from build123d import *

# Parameters (mm, degrees)
SKETCH1_R           = 35
SKETCH1_R_2         = 17.3
BOSS_EXTRUDE1_DEPTH = 2.5
BOSS_EXTRUDE2_START = 2
SKETCH3_R           = 35
SKETCH3_R_2         = 18.6
BOSS_EXTRUDE2_DEPTH = 2
BOSS_EXTRUDE3_START = 2
SKETCH4_R           = 35
SKETCH4_R_2         = 22.3
BOSS_EXTRUDE3_DEPTH = 2
CUT_EXTRUDE1_REACH  = 51.922
SKETCH6_R           = 1.3
BOSS_EXTRUDE6_START = -10
SKETCH7_R           = 35
SKETCH7_W           = 54
SKETCH7_H           = 70
BOSS_EXTRUDE6_DEPTH = 10
SKETCH8_W           = 7
SKETCH8_H           = 70
CUT_EXTRUDE3_DEPTH  = 3
CUT_EXTRUDE4_REACH  = 133.476
SKETCH10_R          = 2.8


with BuildPart() as part:
    # Sketch1 → Boss-Extrude1 (new body)
    with BuildSketch(Plane(origin=(0, 0, 0), x_dir=(1, 0, 0), z_dir=(0, 1, 0))):
        with Locations(Location((0, 0, 0), (0, 0, 270))):
            Circle(SKETCH1_R)
        with Locations(Location((0, 0, 0), (0, 0, 270))):
            Circle(SKETCH1_R_2, mode=Mode.SUBTRACT)
    extrude(amount=BOSS_EXTRUDE1_DEPTH)

    # Sketch3 → Boss-Extrude2 (add)
    with BuildSketch(Plane.XZ.offset(BOSS_EXTRUDE2_START)):
        with Locations(Location((0, 0, 0), (0, 0, 270))):
            Circle(SKETCH3_R)
        with Locations(Location((0, 0, 0), (0, 0, 270))):
            Circle(SKETCH3_R_2, mode=Mode.SUBTRACT)
    extrude(amount=-BOSS_EXTRUDE2_DEPTH)

    # Sketch4 → Boss-Extrude3 (add)
    with BuildSketch(Plane.XZ.offset(2).offset(BOSS_EXTRUDE3_START)):
        with Locations(Location((0, 0, 0), (0, 0, 270))):
            Circle(SKETCH4_R)
        with Locations(Location((0, 0, 0), (0, 0, 270))):
            Circle(SKETCH4_R_2, mode=Mode.SUBTRACT)
    extrude(amount=-BOSS_EXTRUDE3_DEPTH)

    # Sketch6 → Cut-Extrude1 (cut, up to next)
    with BuildSketch(Plane(origin=(0, 2.5, 0), x_dir=(1, 0, 0), z_dir=(0, 1, 0)), mode=Mode.PRIVATE) as cut_extrude1_sk1:
        with Locations(Location((0, 20.25, 0), (0, 0, 270))):
            Circle(SKETCH6_R)
    cut_extrude1_tool1 = extrude(cut_extrude1_sk1.sketch, amount=-CUT_EXTRUDE1_REACH, mode=Mode.PRIVATE) & part.part
    # Sketch6 → Cut-Extrude1 (cut, up to next)
    with BuildSketch(Plane(origin=(0, 2.5, 0), x_dir=(1, 0, 0), z_dir=(0, 1, 0)), mode=Mode.PRIVATE) as cut_extrude1_sk2:
        with Locations(Location((14.318912319, 14.318912319, 0), (0, 0, 270))):
            Circle(SKETCH6_R)
    cut_extrude1_tool2 = extrude(cut_extrude1_sk2.sketch, amount=-CUT_EXTRUDE1_REACH, mode=Mode.PRIVATE) & part.part
    # Sketch6 → Cut-Extrude1 (cut, up to next)
    with BuildSketch(Plane(origin=(0, 2.5, 0), x_dir=(1, 0, 0), z_dir=(0, 1, 0)), mode=Mode.PRIVATE) as cut_extrude1_sk3:
        with Locations(Location((20.25, 0, 0), (0, 0, 270))):
            Circle(SKETCH6_R)
    cut_extrude1_tool3 = extrude(cut_extrude1_sk3.sketch, amount=-CUT_EXTRUDE1_REACH, mode=Mode.PRIVATE) & part.part
    # Sketch6 → Cut-Extrude1 (cut, up to next)
    with BuildSketch(Plane(origin=(0, 2.5, 0), x_dir=(1, 0, 0), z_dir=(0, 1, 0)), mode=Mode.PRIVATE) as cut_extrude1_sk4:
        with Locations(Location((14.318912319, -14.318912319, 0), (0, 0, 270))):
            Circle(SKETCH6_R)
    cut_extrude1_tool4 = extrude(cut_extrude1_sk4.sketch, amount=-CUT_EXTRUDE1_REACH, mode=Mode.PRIVATE) & part.part
    # Sketch6 → Cut-Extrude1 (cut, up to next)
    with BuildSketch(Plane(origin=(0, 2.5, 0), x_dir=(1, 0, 0), z_dir=(0, 1, 0)), mode=Mode.PRIVATE) as cut_extrude1_sk5:
        with Locations(Location((0, -20.25, 0), (0, 0, 270))):
            Circle(SKETCH6_R)
    cut_extrude1_tool5 = extrude(cut_extrude1_sk5.sketch, amount=-CUT_EXTRUDE1_REACH, mode=Mode.PRIVATE) & part.part
    # Sketch6 → Cut-Extrude1 (cut, up to next)
    with BuildSketch(Plane(origin=(0, 2.5, 0), x_dir=(1, 0, 0), z_dir=(0, 1, 0)), mode=Mode.PRIVATE) as cut_extrude1_sk6:
        with Locations(Location((-14.318912319, -14.318912319, 0), (0, 0, 270))):
            Circle(SKETCH6_R)
    cut_extrude1_tool6 = extrude(cut_extrude1_sk6.sketch, amount=-CUT_EXTRUDE1_REACH, mode=Mode.PRIVATE) & part.part
    # Sketch6 → Cut-Extrude1 (cut, up to next)
    with BuildSketch(Plane(origin=(0, 2.5, 0), x_dir=(1, 0, 0), z_dir=(0, 1, 0)), mode=Mode.PRIVATE) as cut_extrude1_sk7:
        with Locations(Location((-20.25, 0, 0), (0, 0, 270))):
            Circle(SKETCH6_R)
    cut_extrude1_tool7 = extrude(cut_extrude1_sk7.sketch, amount=-CUT_EXTRUDE1_REACH, mode=Mode.PRIVATE) & part.part
    # Sketch6 → Cut-Extrude1 (cut, up to next)
    with BuildSketch(Plane(origin=(0, 2.5, 0), x_dir=(1, 0, 0), z_dir=(0, 1, 0)), mode=Mode.PRIVATE) as cut_extrude1_sk8:
        with Locations(Location((-14.318912319, 14.318912319, 0), (0, 0, 270))):
            Circle(SKETCH6_R)
    cut_extrude1_tool8 = extrude(cut_extrude1_sk8.sketch, amount=-CUT_EXTRUDE1_REACH, mode=Mode.PRIVATE) & part.part
    add(cut_extrude1_tool1.solids().sort_by_distance((0, 2.5, -20.25))[0], mode=Mode.SUBTRACT)
    add(cut_extrude1_tool2.solids().sort_by_distance((14.318912, 2.5, -14.318912))[0], mode=Mode.SUBTRACT)
    add(cut_extrude1_tool3.solids().sort_by_distance((20.25, 2.5, 0))[0], mode=Mode.SUBTRACT)
    add(cut_extrude1_tool4.solids().sort_by_distance((14.318912, 2.5, 14.318912))[0], mode=Mode.SUBTRACT)
    add(cut_extrude1_tool5.solids().sort_by_distance((0, 2.5, 20.25))[0], mode=Mode.SUBTRACT)
    add(cut_extrude1_tool6.solids().sort_by_distance((-14.318912, 2.5, 14.318912))[0], mode=Mode.SUBTRACT)
    add(cut_extrude1_tool7.solids().sort_by_distance((-20.25, 2.5, 0))[0], mode=Mode.SUBTRACT)
    add(cut_extrude1_tool8.solids().sort_by_distance((-14.318912, 2.5, -14.318912))[0], mode=Mode.SUBTRACT)

    # Sketch7 → Boss-Extrude6 (add)
    with BuildSketch(Plane(origin=(0, 2.5, 0), x_dir=(1, 0, 0), z_dir=(0, 1, 0)).offset(BOSS_EXTRUDE6_START)):
        Polygon((-45, 55), (99, 55), (119, 55), (119, -55), (99, -55), (-35, -55), (-45, -55), (-45, 35), align=None)
        with Locations(Location((0, 0, 0), (0, 0, 270))):
            Circle(SKETCH7_R, mode=Mode.SUBTRACT)
        with Locations((72, 0)):
            Rectangle(SKETCH7_W, SKETCH7_H, mode=Mode.SUBTRACT)
    extrude(amount=BOSS_EXTRUDE6_DEPTH)

    # Sketch8 → Cut-Extrude3 (cut)
    with BuildSketch(Plane.XZ.offset(7.5)):
        with Locations((102.5, 0)):
            Rectangle(SKETCH8_W, SKETCH8_H)
        with Locations((41.5, 0)):
            Rectangle(SKETCH8_W, SKETCH8_H)
    extrude(amount=-CUT_EXTRUDE3_DEPTH, mode=Mode.SUBTRACT)

    # Sketch10 → Cut-Extrude4 (cut, up to next)
    with BuildSketch(Plane(origin=(0, 2.5, 0), x_dir=(1, 0, 0), z_dir=(0, 1, 0)), mode=Mode.PRIVATE) as cut_extrude4_sk1:
        with Locations(Location((37, 45, 0), (0, 0, 270))):
            Circle(SKETCH10_R)
    cut_extrude4_tool1 = extrude(cut_extrude4_sk1.sketch, amount=-CUT_EXTRUDE4_REACH, mode=Mode.PRIVATE) & part.part
    # Sketch10 → Cut-Extrude4 (cut, up to next)
    with BuildSketch(Plane(origin=(0, 2.5, 0), x_dir=(1, 0, 0), z_dir=(0, 1, 0)), mode=Mode.PRIVATE) as cut_extrude4_sk2:
        with Locations(Location((-35, 45, 0), (0, 0, 270))):
            Circle(SKETCH10_R)
    cut_extrude4_tool2 = extrude(cut_extrude4_sk2.sketch, amount=-CUT_EXTRUDE4_REACH, mode=Mode.PRIVATE) & part.part
    # Sketch10 → Cut-Extrude4 (cut, up to next)
    with BuildSketch(Plane(origin=(0, 2.5, 0), x_dir=(1, 0, 0), z_dir=(0, 1, 0)), mode=Mode.PRIVATE) as cut_extrude4_sk3:
        with Locations(Location((-35, -45, 0), (0, 0, 270))):
            Circle(SKETCH10_R)
    cut_extrude4_tool3 = extrude(cut_extrude4_sk3.sketch, amount=-CUT_EXTRUDE4_REACH, mode=Mode.PRIVATE) & part.part
    # Sketch10 → Cut-Extrude4 (cut, up to next)
    with BuildSketch(Plane(origin=(0, 2.5, 0), x_dir=(1, 0, 0), z_dir=(0, 1, 0)), mode=Mode.PRIVATE) as cut_extrude4_sk4:
        with Locations(Location((37, -45, 0), (0, 0, 270))):
            Circle(SKETCH10_R)
    cut_extrude4_tool4 = extrude(cut_extrude4_sk4.sketch, amount=-CUT_EXTRUDE4_REACH, mode=Mode.PRIVATE) & part.part
    # Sketch10 → Cut-Extrude4 (cut, up to next)
    with BuildSketch(Plane(origin=(0, 2.5, 0), x_dir=(1, 0, 0), z_dir=(0, 1, 0)), mode=Mode.PRIVATE) as cut_extrude4_sk5:
        with Locations(Location((109, 45, 0), (0, 0, 270))):
            Circle(SKETCH10_R)
    cut_extrude4_tool5 = extrude(cut_extrude4_sk5.sketch, amount=-CUT_EXTRUDE4_REACH, mode=Mode.PRIVATE) & part.part
    # Sketch10 → Cut-Extrude4 (cut, up to next)
    with BuildSketch(Plane(origin=(0, 2.5, 0), x_dir=(1, 0, 0), z_dir=(0, 1, 0)), mode=Mode.PRIVATE) as cut_extrude4_sk6:
        with Locations(Location((109, -45, 0), (0, 0, 270))):
            Circle(SKETCH10_R)
    cut_extrude4_tool6 = extrude(cut_extrude4_sk6.sketch, amount=-CUT_EXTRUDE4_REACH, mode=Mode.PRIVATE) & part.part
    # Sketch10 → Cut-Extrude4 (cut, up to next)
    with BuildSketch(Plane(origin=(0, 2.5, 0), x_dir=(1, 0, 0), z_dir=(0, 1, 0)), mode=Mode.PRIVATE) as cut_extrude4_sk7:
        with Locations(Location((109, 0, 0), (0, 0, 270))):
            Circle(SKETCH10_R)
    cut_extrude4_tool7 = extrude(cut_extrude4_sk7.sketch, amount=-CUT_EXTRUDE4_REACH, mode=Mode.PRIVATE) & part.part
    add(cut_extrude4_tool1.solids().sort_by_distance((37, 2.5, -45))[0], mode=Mode.SUBTRACT)
    add(cut_extrude4_tool2.solids().sort_by_distance((-35, 2.5, -45))[0], mode=Mode.SUBTRACT)
    add(cut_extrude4_tool3.solids().sort_by_distance((-35, 2.5, 45))[0], mode=Mode.SUBTRACT)
    add(cut_extrude4_tool4.solids().sort_by_distance((37, 2.5, 45))[0], mode=Mode.SUBTRACT)
    add(cut_extrude4_tool5.solids().sort_by_distance((109, 2.5, -45))[0], mode=Mode.SUBTRACT)
    add(cut_extrude4_tool6.solids().sort_by_distance((109, 2.5, 45))[0], mode=Mode.SUBTRACT)
    add(cut_extrude4_tool7.solids().sort_by_distance((109, 2.5, 0))[0], mode=Mode.SUBTRACT)


solid = part.part
Design review of the part built by this model. Coordinates are the model's own, in mm. A direction names the side the tool comes from. Round coordinates to 2 decimals unless told otherwise and drop trailing zeros. Write each loop counter-clockwise with the first axis right and the second up, starting at its lowest first coordinate (ties: lowest second). Pieces come first, ordered by that corner, then holes. Notation, with made-up numbers: (53, -29.75) - (73, -29.75) arc R17 cw to (73, -24.75) - close; hole circle Ø6 at (89.25, 43.5). An arc over 180 degrees is marked (long way). Use a Markdown table: item, result. Add a question column.
1. We need section C-C (z = 26.5). State the section outline as (x, y) points.
2. Clearance check with flat-ended pins moving along their axes: pin 1 (5.5 mm diameter, centred on x = 102.5, z = 8.5, fed in from -Y); pin 2 (1.5 mm diameter, centred on x = 30.5, z = -14.5, fed in from -Y); pin 3 (4 mm diameter, centred on x = 14.32, z = 14.32, fed in from -Y). State where each tip first meets the part, or that it passes through.
3. We need section A-A (x = 70.5). State the section outline as (y, z) points.
4. Wall thickness on probe 1 along X at (y, z) = (-2.75, 17); probe 2 along X at (y, z) = (-3.5, -4); probe 3 along Z at (x, y) = (51, -6.75): over which ranges is each line inside the solid? List them lowest first.
5. We need section D-D (x = 42). State the section outline as (y, z) points, then the cut area to 3 significant figures.
6. Mouldability with a two-part tool opening along X and no side actions: class faces 1 (the face through (38, -7.5, -37)), 2 (the face through (-45, -3, -1)), 3 (the face through (41, -4.5, 0)), 4 (the face through (119, -3, -1)) as +X half, -X half, draft (parallel to the pull), parting line (faces both ways), or undercut.
7. For faces 5 (the face through (-21.77, -3.01, 4.83)), 6 (the face through (99, -1, 0)), 7 (the face through (38, -3, -55)), list the 3-axis set-ups (+Z, -Z, +X, -X, +Y, -Y) from which the entire face can be reached by the end or side of a thin tool; tool diameter is ignored.
8. We need section B-B (z = -45). State the section outline as (x, y) points, then the cut area to 3 significant figures.
Output:
| question | item | result |
|---|---|---|
| 1 | outline | (-45, -7.5) - (-22.86, -7.5) - (-22.86, -4) - (22.86, -4) - (22.86, -7.5) - (38, -7.5) - (38, -4.5) - (45, -4.5) - (45, 2.5) - (-45, 2.5) - close; (99, -4.5) - (106, -4.5) - (106, -7.5) - (119, -7.5) - (119, 2.5) - (99, 2.5) - close |
| 2 | pin 1 | stops at y = -4.5 |
| 2 | pin 2 | stops at y = -4 |
| 2 | pin 3 | stops at y = -2 |
| 3 | outline | (-7.5, -55) - (2.5, -55) - (2.5, -35) - (-7.5, -35) - close; (-7.5, 35) - (2.5, 35) - (2.5, 55) - (-7.5, 55) - close |
| 4 | probe 1 | x = -45 to -14.43, 14.43 to 45, 99 to 119 |
| 4 | probe 2 | x = -45 to -21.94, 21.94 to 45, 99 to 119 |
| 4 | probe 3 | z = -55 to -35, 35 to 55 |
| 5 | outline | (-7.5, -55) - (2.5, -55) - (2.5, 55) - (-7.5, 55) - (-7.5, 35) - (-4.5, 35) - (-4.5, -35) - (-7.5, -35) - close |
| 5 | area | 890 mm2 |
| 6 | face 1 | draft |
| 6 | face 2 | -X half |
| 6 | face 3 | undercut |
| 6 | face 4 | +X half |
| 7 | face 5 | -Y |
| 7 | face 6 | +Y, -Y |
| 7 | face 7 | -Z, +X, -X, +Y, -Y |
| 8 | outline | (-45, -7.5) - (-37.8, -7.5) - (-37.8, 2.5) - (-45, 2.5) - close; (-32.2, -7.5) - (34.2, -7.5) - (34.2, 2.5) - (-32.2, 2.5) - close; (39.8, -7.5) - (106.2, -7.5) - (106.2, 2.5) - (39.8, 2.5) - close; (111.8, -7.5) - (119, -7.5) - (119, 2.5) - (111.8, 2.5) - close |
| 8 | area | 1,470 mm2 |
